Read the model definition and answer for the solid it produces. Units are mm, in the model's axes. Coordinates: 2 decimals unless noted, no trailing zeros. Order: outer loops, then holes, each group sorted by start corner. A loop starts at its lowest first (then second) coordinate and runs counter-clockwise, first axis right, second up. Notation, with made-up numbers: (10.25, -39) -> (25.25, -39) arc R23 ccw to (25.25, -21) -> close; hole circle Ø10 at (4, 51). An arc over 180 degrees is marked (long way). Use CSV: the item, a comma, the result in double quotes.
```python
from build123d import *

# Parameters (mm, degrees)
BOSS_EXTRUDE1_DEPTH = 3


with BuildPart() as part:
    # Sketch1 → Boss-Extrude1 (new body)
    with BuildSketch(Plane.XY):
        with BuildLine():
            Line((-307.184555639, 613.714480845), (-347.184555639, 613.714480845))
            ThreePointArc((-347.184555639, 613.714480845), (-348.598769202, 613.128694407), (-349.184555639, 611.714480845))
            Line((-349.184555639, 611.714480845), (-349.184555639, 571.714480845))
            ThreePointArc((-349.184555639, 571.714480845), (-348.598769202, 570.300267282), (-347.184555639, 569.714480845))
            Line((-347.184555639, 569.714480845), (-327.414726928, 569.714480845))
            ThreePointArc((-327.414726928, 569.714480845), (-326.021875182, 570.279223372), (-325.415626051, 571.65451683))
            ThreePointArc((-325.415626051, 571.65451683), (-319.898638459, 584.428563664), (-307.124591625, 589.945551256))
            ThreePointArc((-307.124591625, 589.945551256), (-305.749298166, 590.551800388), (-305.184555639, 591.944652133))
            Line((-305.184555639, 591.944652133), (-305.184555639, 611.714480845))
            ThreePointArc((-305.184555639, 611.714480845), (-305.770342077, 613.128694407), (-307.184555639, 613.714480845))
        make_face()
    extrude(amount=BOSS_EXTRUDE1_DEPTH)


solid = part.part
```
Item 1: Find section A-A, the plane z = 1.15. Give the vertices of the cut face in (x, y), then the cut area to 3 significant figures.
Return value:
outline,"(-349.18, 571.71) arc R2 ccw to (-347.18, 569.71) -> (-327.41, 569.71) arc R2 ccw to (-325.42, 571.65) arc R18.87 cw to (-307.12, 589.95) arc R2 ccw to (-305.18, 591.94) -> (-305.18, 611.71) arc R2 ccw to (-307.18, 613.71) -> (-347.18, 613.71) arc R2 ccw to (-349.18, 611.71) -> close"
area,"1,600 mm^2"
Item 2: Straight lines are drawn through the part: line 1 along Y through (x, z) = (-312.5, 0.8); line 2 along X through (y, z) = (579.5, 2.35); line 3 along X through (y, z) = (584, 1.4). For each, find the intervals that lie inside material, in ascending order.
Return value:
line 1,"y = 588.99 to 613.71"
line 2,"x = -349.18 to -323.45"
line 3,"x = -349.18 to -320.31"
Item 3: Find section B-B, the plane y = 584. Give the vertices of the cut face in (x, z).
Return value:
outline,"(-349.18, 0) -> (-320.31, 0) -> (-320.31, 3) -> (-349.18, 3) -> close"
Item 4: Find section C-C, the plane x = -320. Give the vertices of the cut face in (y, z).
Return value:
outline,"(584.33, 0) -> (613.71, 0) -> (613.71, 3) -> (584.33, 3) -> close"
Item 5: Each of these flat-tipped pins is pushed along its axis until it touches: P1, Ø1.5, axis at x = -338, y = 589, coming from the -Z side; P2, Ø1.5, axis at x = -318, z = 2.5, coming from the -Y side. Where does it stop, or does it pass through?
Return value:
P1,"stops at z = 0"
P2,"stops at y = 585.49"
